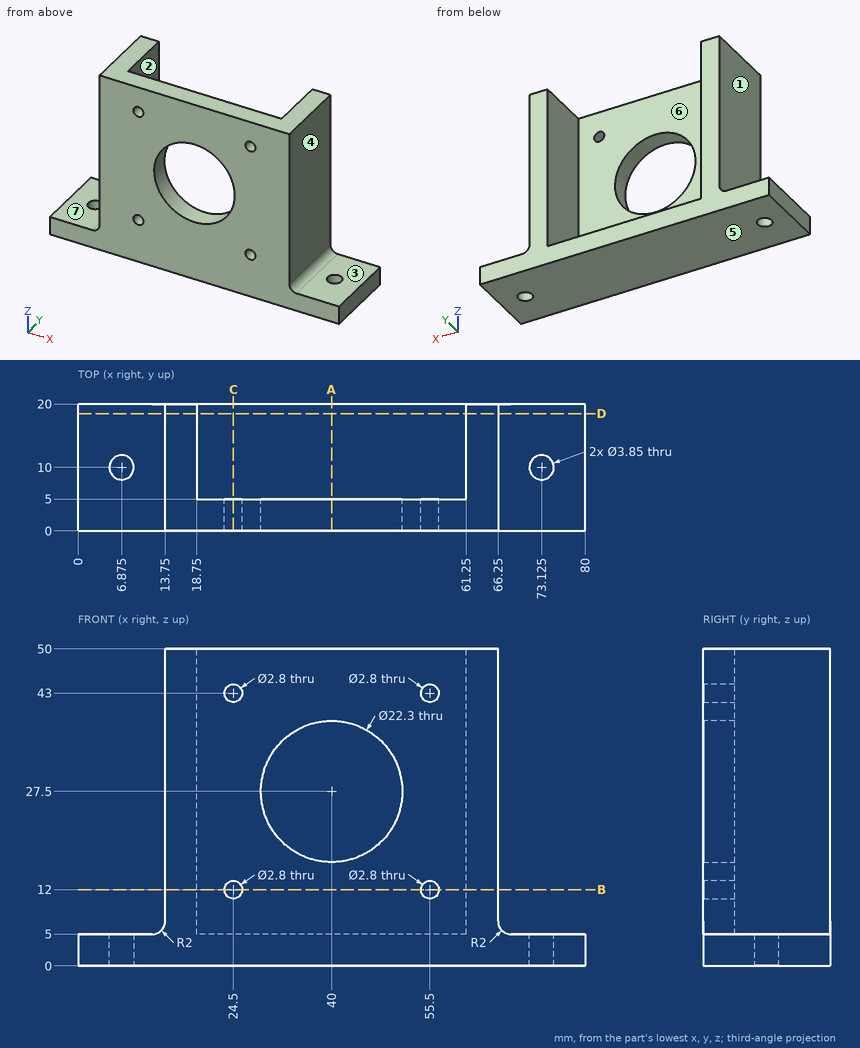
Answer from the drawing. Dimensions are ordinates in mm from the lowest x, y and z of the part. A direction names the side the tool comes from. Give positions to 0.01 mm unless a question says otherwise; leave off trailing zeros. Write each loop counter-clockwise with the first axis right and the second up, starting at its lowest first coordinate (ties: lowest second). Pieces come first, ordered by that corner, then holes. Notation, with made-up numbers: (-4.5, 86.25) - (7.5, 86.25) arc R22 cw to (7.5, 96.25) - close; hole circle Ø8 at (27, 20.5). An arc over 180 degrees is marked (long way). Answer in a Markdown table with one row per item. Add a question column.
Item 1: Find the intervals of material crossed by L1, parallel to X at y = 2.8, z = 27.5; L2, parallel to X at y = 12.75, z = 33; L3, parallel to X at y = 3.75, z = 12, in increasing order.
Item 2: Flat-ended cylindrical pins translate along their axes: P1, Ø7.5, axis at y = 14, z = 26, coming from the +X side; P2, Ø7.5, axis at x = 45.5, y = 14, coming from the +Z side; P3, Ø9.5, axis at x = 71.5, y = 11.5, coming from the +Z side. Find the tip coordinate at first contact, or state that the pin passes through.
Item 3: Section B-B, the plane z = 12 is taken. Write down the section's boundary in (x, y), and give its area (4 significant figures).
Item 4: Section C-C, the plane x = 24.5 is taken. Write down the section's boundary in (y, z).
Item 5: Section D-D, the plane y = 18.5 is taken. Write down the section's boundary in (x, z), and give its area (3 significant figures).
Item 6: A tool of negligible diameter and unlimited length cuts with its end or side. For the marked faces 5, 6 and 7, from which of +Z, -Z, +X, -X, +Y, -Y can it reach the whole face along a straight path? Write none if from no direction.
Item 7: Determine the mould class of the marked faces 1, 2, 3 and 4 for opening direction X: pulls with the +X half, pulls with the -X half, needs draft (parallel to the pull), parting line crosses it, or undercut.
Item 8: Section A-A, the plane x = 40 is taken. Write down the section's boundary in (y, z).
Recorded:
| question | item | result |
|---|---|---|
| 1 | L1 | x = 13.75 to 28.85, 51.15 to 66.25 |
| 1 | L2 | x = 13.75 to 18.75, 61.25 to 66.25 |
| 1 | L3 | x = 13.75 to 23.1, 25.9 to 54.1, 56.9 to 66.25 |
| 2 | P1 | stops at x = 66.25 |
| 2 | P2 | stops at z = 5 |
| 2 | P3 | stops at z = 5.68 |
| 3 | outline | (13.75, 0) - (23.1, 0) - (23.1, 5) - (18.75, 5) - (18.75, 20) - (13.75, 20) - close; (25.9, 0) - (54.1, 0) - (54.1, 5) - (25.9, 5) - close; (56.9, 0) - (66.25, 0) - (66.25, 20) - (61.25, 20) - (61.25, 5) - (56.9, 5) - close |
| 3 | area | 384.5 mm2 |
| 4 | outline | (0, 0) - (20, 0) - (20, 5) - (5, 5) - (5, 10.6) - (0, 10.6) - close; (0, 13.4) - (5, 13.4) - (5, 41.6) - (0, 41.6) - close; (0, 44.4) - (5, 44.4) - (5, 50) - (0, 50) - close |
| 5 | outline | (0, 0) - (80, 0) - (80, 5) - (68.25, 5) arc R2 cw to (66.25, 7) - (66.25, 50) - (61.25, 50) - (61.25, 5) - (18.75, 5) - (18.75, 50) - (13.75, 50) - (13.75, 7) arc R2 cw to (11.75, 5) - (0, 5) - close |
| 5 | area | 852 mm2 |
| 6 | face 5 | -Z, +X, -X, +Y, -Y |
| 6 | face 6 | +Z, +Y |
| 6 | face 7 | +Z, -X, +Y, -Y |
| 7 | face 1 | pulls with the -X half |
| 7 | face 2 | undercut |
| 7 | face 3 | needs draft |
| 7 | face 4 | pulls with the +X half |
| 8 | outline | (0, 0) - (20, 0) - (20, 5) - (5, 5) - (5, 16.35) - (0, 16.35) - close; (0, 38.65) - (5, 38.65) - (5, 50) - (0, 50) - close |
